Input: part model. Units: mm. Frame: model coordinates. Face numbers are marked on the shaded views. A direction names the side the tool comes from. Round coordinates to 2 decimals unless told otherwise and drop trailing zeros. Loops run counter-clockwise (first coordinate to the right, second up) from the corner with the lowest first, then second, coordinate; pieces in that order, holes last. Notation, with made-up numbers: M -19.5,9.25 L 35.5,9.25 A22 cw 35.5,38.25 Z; hole C -21.75,22.25 d11. An arc over 180 degrees is marked long. Return JSON: item names as keys, results as strings. Group by question number.
1) Section C-C (z = 0.9). Count the separate pieces of the cut face and the enclosed holes in it, plus the area to 3 significant figures.
2) Section B-B (x = 150.75). Output: boundary loops of the cut face in (y, z).
3) Section A-A (y = 199.5). Output: boundary loops of the cut face in (x, z), plus the area to 4 significant figures.
4) Access query for the marked faces 1, 2 and 3. Directions: +Z, -Z, +X, -X, +Y, -Y. A direction counts if a zero-diameter tool reaches every point of the face in a straight line with its end or side. Return the directions, or none.
5) Section D-D (y = 208.5). Output: boundary loops of the cut face in (x, z).
6) Material intervals for line 1 (X direction, y = 207.75, z = 0.8); line 2 (Y direction, x = 159.25, z = 0.75); line 3 (X direction, y = 199, z = 2.5), sorted ascending. Write a range as from..to.
7) Contact query for flat-ended pins moving along their axis: P1, Ø1.5, axis at x = 148, y = 208.5, coming from the -Z side; P2, Ø1.5, axis at y = 199.5, z = 1, coming from the -X side; P3, Ø1.5, axis at x = 152.5, z = 1, coming from the -Y side. Output: stop coordinate, or through.
from build123d import *

# Parameters (mm, degrees)
SALIENTE_EXTRUIR1_DEPTH = 3


with BuildPart() as part:
    # Model → Saliente-Extruir1 (new body)
    with BuildSketch(Plane.XY):
        with BuildLine():
            Line((149.34213351, 211.823953209), (158.34213351, 211.823953209))
            Line((158.34213351, 211.823953209), (162.84213351, 211.823953209))
            Line((162.84213351, 211.823953209), (162.84213351, 198.323953209))
            Line((162.84213351, 198.323953209), (162.84213351, 193.823953209))
            Line((162.84213351, 193.823953209), (158.34213351, 193.823953209))
            ThreePointArc((158.34213351, 193.823953209), (155.160152994, 195.141972694), (153.84213351, 198.323953209))
            Line((153.84213351, 198.323953209), (153.84213351, 202.823953209))
            Line((153.84213351, 202.823953209), (149.34213351, 202.823953209))
            ThreePointArc((149.34213351, 202.823953209), (146.160152994, 204.141972694), (144.84213351, 207.323953209))
            Line((144.84213351, 207.323953209), (144.84213351, 211.823953209))
            Line((144.84213351, 211.823953209), (149.34213351, 211.823953209))
        make_face()
        with BuildLine():
            Line((156.71713351, 195.823953209), (156.71713351, 200.823953209))
            ThreePointArc((156.71713351, 200.823953209), (156.936803424, 201.354283295), (157.46713351, 201.573953209))
            Line((157.46713351, 201.573953209), (159.21713351, 201.573953209))
            ThreePointArc((159.21713351, 201.573953209), (159.747463595, 201.354283295), (159.96713351, 200.823953209))
            Line((159.96713351, 200.823953209), (159.96713351, 195.823953209))
            ThreePointArc((159.96713351, 195.823953209), (159.747463595, 195.293623123), (159.21713351, 195.073953209))
            Line((159.21713351, 195.073953209), (157.46713351, 195.073953209))
            ThreePointArc((157.46713351, 195.073953209), (156.936803424, 195.293623123), (156.71713351, 195.823953209))
        make_face(mode=Mode.SUBTRACT)
        with BuildLine():
            Line((151.84213351, 205.698953209), (146.84213351, 205.698953209))
            ThreePointArc((146.84213351, 205.698953209), (146.311803424, 205.918623123), (146.09213351, 206.448953209))
            Line((146.09213351, 206.448953209), (146.09213351, 208.198953209))
            ThreePointArc((146.09213351, 208.198953209), (146.311803424, 208.729283295), (146.84213351, 208.948953209))
            Line((146.84213351, 208.948953209), (151.84213351, 208.948953209))
            ThreePointArc((151.84213351, 208.948953209), (152.372463595, 208.729283295), (152.59213351, 208.198953209))
            Line((152.59213351, 208.198953209), (152.59213351, 206.448953209))
            ThreePointArc((152.59213351, 206.448953209), (152.372463595, 205.918623123), (151.84213351, 205.698953209))
        make_face(mode=Mode.SUBTRACT)
        with BuildLine():
            Line((160.84213351, 205.698953209), (155.84213351, 205.698953209))
            ThreePointArc((155.84213351, 205.698953209), (155.311803424, 205.918623123), (155.09213351, 206.448953209))
            Line((155.09213351, 206.448953209), (155.09213351, 208.198953209))
            ThreePointArc((155.09213351, 208.198953209), (155.311803424, 208.729283295), (155.84213351, 208.948953209))
            Line((155.84213351, 208.948953209), (160.84213351, 208.948953209))
            ThreePointArc((160.84213351, 208.948953209), (161.372463595, 208.729283295), (161.59213351, 208.198953209))
            Line((161.59213351, 208.198953209), (161.59213351, 206.448953209))
            ThreePointArc((161.59213351, 206.448953209), (161.372463595, 205.918623123), (160.84213351, 205.698953209))
        make_face(mode=Mode.SUBTRACT)
    extrude(amount=SALIENTE_EXTRUIR1_DEPTH)


solid = part.part
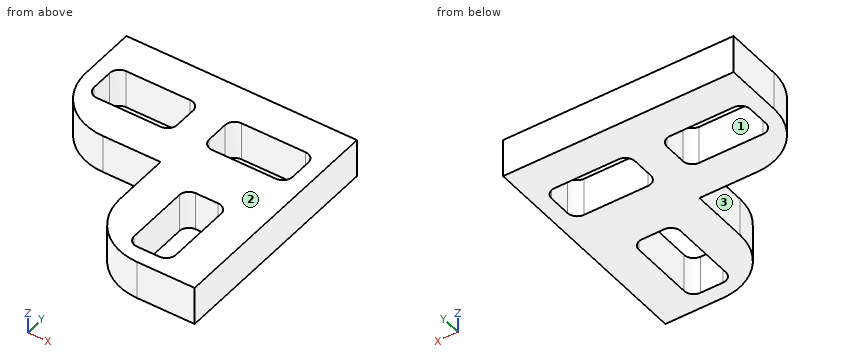
Returned:
{
 "1": {"separate pieces": "1", "enclosed holes": "3", "area": "172 mm^2"},
 "2": {"outline": "M 202.82,0 L 205.7,0 L 205.7,3 L 202.82,3 Z; M 208.95,0 L 211.82,0 L 211.82,3 L 208.95,3 Z"},
 "3": {"outline": "M 153.84,0 L 156.72,0 L 156.72,3 L 153.84,3 Z; M 159.97,0 L 162.84,0 L 162.84,3 L 159.97,3 Z", "area": "17.25 mm^2"},
 "4": {"face 1": "+Z, -Z", "face 2": "+Z, +X, -X, +Y, -Y", "face 3": "+Z, -Z, -X, -Y"},
 "5": {"outline": "M 144.84,0 L 146.16,0 L 146.16,3 L 144.84,3 Z; M 152.53,0 L 155.16,0 L 155.16,3 L 152.53,3 Z; M 161.53,0 L 162.84,0 L 162.84,3 L 161.53,3 Z"},
 "6": {"line 1": "x = 144.84..146.09, 152.59..155.09, 161.59..162.84", "line 2": "y = 193.82..195.07, 201.57..205.7, 208.95..211.82", "line 3": "x = 153.84..156.72, 159.97..162.84"},
 "7": {"P1": "stops at z = 0", "P2": "stops at x = 153.84", "P3": "stops at y = 202.82"}
}
